from build123d import *

# Parameters (mm, degrees)
SKETCH20_W                     = 61.5
SKETCH20_H                     = 17
BASE_FLANGE1_DEPTH             = 3.048
EDGE_FLANGE1_STRIP_W           = 15.24
EDGE_FLANGE1_STRIP_H           = 3.048
EDGE_FLANGE1_STRIP_CUT_DEPTH   = 17
EDGE_FLANGE1_STRIP_2_W         = 15.24
EDGE_FLANGE1_STRIP_2_H         = 3.048
EDGE_FLANGE1_STRIP_CUT_2_DEPTH = 17
EDGE_FLANGE1_DEPTH             = 17
EDGE_FLANGE1_BEND_DEPTH        = 17
CUT_EXTRUDE3_DEPTH             = 66.770177923
CUT_EXTRUDE3_DEPTH_BACK        = 66.770177923
M3_CLEARANCE_HOLE1_D           = 3.4


# Sheet-metal steps are written as plain solids
with BuildPart() as part:
    # Sketch20 → Base-Flange1 (new body)
    with BuildSketch(Plane(origin=(0, 0, 0), x_dir=(1, 0, 0), z_dir=(0, 1, 0))):
        with Locations((30.75, 8.5)):
            Rectangle(SKETCH20_W, SKETCH20_H)
    extrude(amount=-BASE_FLANGE1_DEPTH)

    # Edge-Flange1 strip (across the edge) → Edge-Flange1 strip cut (cut)
    with BuildSketch(Plane.XY.offset(-17)):
        with Locations((-3.048, -1.524)):
            Rectangle(EDGE_FLANGE1_STRIP_W, EDGE_FLANGE1_STRIP_H)
    extrude(amount=EDGE_FLANGE1_STRIP_CUT_DEPTH, mode=Mode.SUBTRACT)

    # Edge-Flange1 strip 2 (across the edge) → Edge-Flange1 strip cut 2 (cut)
    with BuildSketch(Plane(origin=(61.5, 0, 0), x_dir=(-1, 0, 0), z_dir=(0, 0, -1))):
        with Locations((-3.048, -1.524)):
            Rectangle(EDGE_FLANGE1_STRIP_2_W, EDGE_FLANGE1_STRIP_2_H)
    extrude(amount=EDGE_FLANGE1_STRIP_CUT_2_DEPTH, mode=Mode.SUBTRACT)

    # Edge-Flange1 section (across the edge) → Edge-Flange1 (add)
    with BuildSketch(Plane.XY.offset(-17)):
        with BuildLine():
            Line((0, 1.524), (0, 15.952))
            Line((0, 15.952), (3.048, 15.952))
            Line((3.048, 15.952), (3.048, 1.524))
            ThreePointArc((3.048, 1.524), (3.494369265, 0.446369265), (4.572, 0))
            Line((4.572, 0), (4.572, -3.048))
            ThreePointArc((4.572, -3.048), (1.339107796, -1.708892204), (0, 1.524))
        make_face()
    extrude(amount=EDGE_FLANGE1_DEPTH)

    # Edge-Flange1 section 2 (across the edge) → Edge-Flange1 bend (add)
    with BuildSketch(Plane(origin=(61.5, 0, 0), x_dir=(-1, 0, 0), z_dir=(0, 0, -1))):
        with BuildLine():
            Line((0, 1.524), (0, 15.952))
            Line((0, 15.952), (3.048, 15.952))
            Line((3.048, 15.952), (3.048, 1.524))
            ThreePointArc((3.048, 1.524), (3.494369265, 0.446369265), (4.572, 0))
            Line((4.572, 0), (4.572, -3.048))
            ThreePointArc((4.572, -3.048), (1.339107796, -1.708892204), (0, 1.524))
        make_face()
    extrude(amount=EDGE_FLANGE1_BEND_DEPTH)

    # Sketch29 → Cut-Extrude3 (cut, two sides: drawn at the far end of the back side and taken through both)
    with BuildSketch(Plane(origin=(0, 0, 0), x_dir=(0, 0, -1), z_dir=(1, 0, 0)).offset(-CUT_EXTRUDE3_DEPTH_BACK)):
        with BuildLine():
            Line((0, 1.524), (0, 2.594))
            ThreePointArc((0, 2.594), (0.210525003, 3.698005998), (0.812552829, 4.647064751))
            Line((0.812552829, 4.647064751), (3.562552829, 7.577064751))
            ThreePointArc((3.562552829, 7.577064751), (4.558193441, 8.277106814), (5.75, 8.524))
            Line((5.75, 8.524), (11.25, 8.524))
            ThreePointArc((11.25, 8.524), (12.441806559, 8.277106814), (13.437447171, 7.577064751))
            Line((13.437447171, 7.577064751), (16.187447171, 4.647064751))
            ThreePointArc((16.187447171, 4.647064751), (16.789474997, 3.698005998), (17, 2.594))
            Line((17, 2.594), (17, 1.524))
            Line((17, 1.524), (21.797856885, 1.524))
            Line((21.797856885, 1.524), (21.797856885, 17.003274098))
            Line((21.797856885, 17.003274098), (-4.797856885, 17.003274098))
            Line((-4.797856885, 17.003274098), (-4.797856885, 1.524))
            Line((-4.797856885, 1.524), (0, 1.524))
        make_face()
    extrude(amount=CUT_EXTRUDE3_DEPTH + CUT_EXTRUDE3_DEPTH_BACK, mode=Mode.SUBTRACT)

    # M3 Clearance Hole1 (through all)
    with Locations(Plane(origin=(0, 4.524, -13.05), x_dir=(0, -1, 0), z_dir=(-1, 0, 0))):
        with Locations((0, 0), (0, 6.6)):
            Hole(M3_CLEARANCE_HOLE1_D / 2)


solid = part.part
Input: part model. Units: mm. Frame: model coordinates. Coordinates: 2 decimals unless noted, no trailing zeros. Loops run counter-clockwise (first coordinate to the right, second up) from the corner with the lowest first, then second, coordinate; pieces in that order, holes last. Notation, with made-up numbers: (-30, 20) -> (-21, 20) arc R35 ccw to (-21, 59) -> close; hole circle Ø6 at (-17, -3). An arc over 180 degrees is marked (long way). Write each question's results on one line, items separated by ' | '. Start each with the question number.
Q1. Section C-C, the plane x = 41. Return the cut outline in (y, z).
Q2. Pin query (flat end, axial travel): pin 1 (5 mm diameter, centred on x = 26.5, z = -7.5, fed in from +Y). Return the tip coordinate at first contact, or that it passes through.
Q3. Section A-A, the plane z = -6.45. Return the cut outline in (x, y), plus the area to 3 significant figures.
Q4. Section B-B, the plane y = 7. Return the cut outline in (x, z), plus the area to 3 significant figures.
Q5. Ray query, line 1 (X direction, y = 2.5, z = -2.5); line 2 (Z direction, x = 59.5, y = 3.5); line 3 (Y direction, x = 14, z = -15.5). Return the intervals inside material, ascending. Write a range as from..to.
Q6. Pull-direction query (X, two-part tool) for faces 1 (the flat face through (58.452, 4.3, -8.4)), 2 (the flat face through (61.5, 4.2, -8.4)), 3 (the cylindrical face through (3.48, 0.46, -8.62)), 4 (the flat face through (30, -1, -17)); classes: released by +X, released by -X, zero draft, split by the parting line, or undercut.
Found:
1) outline: (-3.05, -17) -> (0, -17) -> (0, 0) -> (-3.05, 0) -> close
2) pin 1: y = 0
3) outline: (0, 1.52) arc R4.57 ccw to (4.57, -3.05) -> (56.93, -3.05) arc R4.57 ccw to (61.5, 1.52) -> (61.5, 2.82) -> (58.45, 2.82) -> (58.45, 1.52) arc R1.52 cw to (56.93, 0) -> (4.57, 0) arc R1.52 cw to (3.05, 1.52) -> (3.05, 2.82) -> (0, 2.82) -> close; (0, 6.22) -> (3.05, 6.22) -> (3.05, 8.52) -> (0, 8.52) -> close; (58.45, 6.22) -> (61.5, 6.22) -> (61.5, 8.52) -> (58.45, 8.52) -> close | area: 211 mm2
4) outline: (0, -13.98) -> (3.05, -13.98) -> (3.05, -3.02) -> (0, -3.02) -> close; (58.45, -13.98) -> (61.5, -13.98) -> (61.5, -3.02) -> (58.45, -3.02) -> close | area: 66.8 mm2
5) line 1: 0..3.05, 58.45..61.5 | line 2: -16.86..-14.41, -11.69..-7.81, -5.09..-0.14 | line 3: -3.05..0
6) face 1: undercut | face 2: released by +X | face 3: undercut | face 4: zero draft
